Verification items for the finished model (mm, model axes). A direction names the side the tool comes from. Give positions to 0.01 mm unless a question says otherwise; leave off trailing zeros. Write each loop counter-clockwise with the first axis right and the second up, starting at its lowest first coordinate (ties: lowest second). Pieces come first, ordered by that corner, then holes. Notation, with made-up numbers: M 7.25,32.5 L 16.25,32.5 A9 ccw 16.25,47.5 Z; hole C -22.5,-4 d10. An arc over 180 degrees is marked long. Answer as a JSON object with one key per item and string values.
```python
from build123d import *

# Parameters (mm, degrees)
SKETCH1_W               = 94
SKETCH1_H               = 8.9
BOSS_EXTRUDE1_DEPTH     = 6
BOSS_EXTRUDE2_DEPTH     = 10
FILLET1_R               = 1
CUT_EXTRUDE1_DEPTH      = 113.775218909
CUT_EXTRUDE1_DEPTH_BACK = 113.775218909
SKETCH3_W               = 150
SKETCH3_H               = 7


with BuildPart() as part:
    # Sketch1 → Boss-Extrude1 (new body)
    with BuildSketch(Plane(origin=(0, 0, 0), x_dir=(1, 0, 0), z_dir=(0, 1, 0))):
        Polygon((106.5, 2.9), (106.5, 5.15), (108.9, 5.15), (108.9, -2.25), (106.5, -2.25), (106.5, 0), (81.5, 0), (81.5, -6), (-18.5, -6), (-18.5, -0.05), (-48.5, -0.05), (-48.5, -6), (-68.5, -6), (-68.5, 0), (-108.8, 0), (-108.8, -2.25), (-111.2, -2.25), (-111.2, 5.15), (-108.8, 5.15), (-108.8, 2.9), (-68.5, 2.9), (-68.5, 8.9), (-48.5, 8.9), (-48.5, 2.95), (-18.5, 2.95), (-18.5, 8.9), (81.5, 8.9), (81.5, 2.9), align=None)
        with Locations((31.5, 1.45)):
            Rectangle(SKETCH1_W, SKETCH1_H, mode=Mode.SUBTRACT)
    extrude(amount=BOSS_EXTRUDE1_DEPTH)

    # Sketch2 → Boss-Extrude2 (add)
    with BuildSketch(Plane(origin=(0, 6, 0), x_dir=(1, 0, 0), z_dir=(0, 1, 0))):
        Polygon((-65.9, 6.9), (-65.9, 15.9), (-63.9, 15.9), (-63.9, 8.9), (-56.9, 8.9), (-56.9, 6.9), align=None)
        Polygon((-65.9, -4), (-56.9, -4), (-56.9, -6), (-63.9, -6), (-63.9, -13), (-65.9, -13), align=None)
        Polygon((65.9, -13), (65.9, -4), (56.9, -4), (56.9, -6), (63.9, -6), (63.9, -13), align=None)
        Polygon((56.9, 6.9), (65.9, 6.9), (65.9, 15.9), (63.9, 15.9), (63.9, 8.9), (56.9, 8.9), align=None)
    extrude(amount=-BOSS_EXTRUDE2_DEPTH)

    # Fillet1
    fillet1_edges = [part.edges().sort_by_distance(p)[0] for p in [
        (-68.5, 0, 3),
        (-68.5, 0, -5.9),
        (-108.8, 0, -4.025),
        (-108.8, 0, 1.125),
        (-68.5, 3, 0),
        (-68.5, 3, -2.9),
        (-88.65, 0, 0),
        (-88.65, 0, -2.9),
        (81.5, 0, -5.9),
        (81.5, 0, 3),
        (78.5, 3, -5.9),
        (78.5, 3, 3),
        (-15.5, 3, 3),
        (-15.5, 3, -5.9),
        (-18.5, 3, -2.95),
        (-18.5, 3, 0.05),
        (-48.5, 3, -2.95),
        (-48.5, 3, 0.05),
        (-65.9, 3, 6),
        (-65.9, 3, -8.9),
        (65.9, 3, -8.9),
        (65.9, 3, 6),
        (81.5, 3, -2.9),
        (81.5, 3, 0),
        (106.5, 0, 1.125),
        (107.7, 0, 2.25),
        (108.9, 0, -1.45),
        (107.7, 0, -5.15),
        (106.5, 0, -4.025),
        (94, 0, -2.9),
        (94, 0, 0),
    ]]
    fillet(fillet1_edges, radius=FILLET1_R)

    # Sketch3 → Cut-Extrude1 (cut, two sides: drawn at the far end of the back side and taken through both)
    with BuildSketch(Plane(origin=(0, 6, 0), x_dir=(1, 0, 0), z_dir=(0, 1, 0)).offset(-CUT_EXTRUDE1_DEPTH_BACK)):
        with Locations((6.5, -9.5)):
            Rectangle(SKETCH3_W, SKETCH3_H)
    extrude(amount=CUT_EXTRUDE1_DEPTH + CUT_EXTRUDE1_DEPTH_BACK, mode=Mode.SUBTRACT)


solid = part.part
```
1) Section check C-C on x = 89. Record the boundary of the cut face in (y, z), and give its area (3 significant figures).
Completed:
{"outline": "M 0,-1.9 A1 ccw 1,-2.9 L 6,-2.9 L 6,0 L 1,0 A1 ccw 0,-1 Z", "area": "17.0 mm2"}
2) Access from +Z, -Z, +X, -X, +Y, -Y to the whole of each face (thin tool, end or side, straight path). Record for faces 4 (the face through (-48.5, 3, 3)), 5 (the face through (22, 3, -8.9)), 6 (the face through (74, 3, -8.9)), 7 (the face through (-15.5, 3, -1)).
Completed:
{"face 4": "+Z, +Y, -Y", "face 5": "-Z, +Y, -Y", "face 6": "-Z, +X, +Y, -Y", "face 7": "+Y, -Y"}
3) Section check A-A on z = -11.75. Record the boundary of the cut face in (x, y), and give its area (3 significant figures).
Completed:
{"outline": "M -65.9,-4 L -63.9,-4 L -63.9,6 L -65.9,6 Z; M 63.9,-4 L 65.9,-4 L 65.9,6 L 63.9,6 Z", "area": "40.0 mm2"}
4) Go/stop test with flat-tipped pins: pin 1 (4 mm diameter, centred on x = -27, y = -0.5, fed in from -Z); pin 2 (2.5 mm diameter, centred on y = 3.5, z = 4.5, fed in from -X); pin 3 (4.5 mm diameter, centred on y = 1.5, z = -11.5, fed in from +X); pin 4 (5.5 mm diameter, centred on y = 2.5, z = 4.5, fed in from +X). Record where each tip stops, or that it passes through.
Completed:
{"pin 1": "stops at z = -2.95", "pin 2": "stops at x = -68.5", "pin 3": "stops at x = 66.14", "pin 4": "stops at x = 108.9"}
5) Release check for a two-part mould opening along Z. For faces 1 (the face through (-48.5, 3, -6)), 2 (the face through (-58, 2, 6)), 3 (the face through (78.5, 3, -1)) record: pulls with the +Z half, pulls with the -Z half, needs draft (parallel to the pull), parting line crosses it, or undercut.
Completed:
{"face 1": "needs draft", "face 2": "pulls with the +Z half", "face 3": "undercut"}
6) Thickness scan on L1, parallel to X at y = 5, z = -4; L2, parallel to X at y = 5.75, z = -1; L3, parallel to Z at x = 26, y = 1.75. Record the ranges inside material, lowest first.
Completed:
{"L1": "x = -111.2 to -108.8, -68.5 to -48.5, -18.5 to -15.5, 78.5 to 81.5, 106.5 to 108.9", "L2": "x = -111.2 to -15.5, 78.5 to 108.9", "L3": "z = -8.9 to -5.9, 3 to 6"}
7) Section check B-B on x = -12. Record the boundary of the cut face in (y, z).
Completed:
{"outline": "M 0,-8.9 L 6,-8.9 L 6,-5.9 L 0,-5.9 Z; M 0,3 L 6,3 L 6,6 L 0,6 Z"}
8) Section check D-D on x = -42.5. Record the boundary of the cut face in (y, z), and give its area (3 significant figures).
Completed:
{"outline": "M 0,-2.95 L 6,-2.95 L 6,0.05 L 0,0.05 Z", "area": "18.0 mm2"}
